Model file for the job. Use its own axes, mm. A direction names the side the tool comes from. Round coordinates to 2 decimals unless told otherwise and drop trailing zeros. Order: outer loops, then holes, each group sorted by start corner. A loop starts at its lowest first (then second) coordinate and runs counter-clockwise, first axis right, second up. Notation, with made-up numbers: M -2.75,85 L 38.25,85 A33 cw 38.25,119 Z; hole C 82.5,14 d2. An arc over 180 degrees is marked long. Return JSON: item names as keys, results as strings. Group by question number.
Item 1: Slice it at C-C on y = 9.75. Write the cut outline in (x, z), then the cut area to 3 significant figures.
Item 2: Pull direction X, two halves, no side cores. Call faces 1 (the face through (-1.743, 8.765, 1.901)), 2 (the face through (-7.374, 6.383, 2.322)), 3 (the face through (2, 11.112, 2)): pulls with the +X half, pulls with the -X half, needs draft (parallel to the pull), parting line crosses it, or undercut.
Item 3: Pin check, flat tips, straight feed: pin 1 Ø6 at (y, z) = (5, -4.5) entering from +X; pin 2 Ø4 at (x, z) = (0, -1) entering from -Y; pin 3 Ø6 at (x, y) = (-4.5, 2) entering from -Z. Stop position of each tip, or through.
Item 4: Slice it at D-D on y = 1.25. Write the cut outline in (x, z), then the cut area to 3 significant figures.
Item 5: Probe line 1 along X through (y, z) = (3.25, -2.75); line 2 along Z through (x, y) = (0, 7.55); line 3 along Y through (x, z) = (2.5, 2.5). List the from-to ranges inside material, lowest first.
Item 6: Which spindle directions (+Z, -Z, +X, -X, +Y, -Y) get a long thin tool onto all of the face, cutting with end or side? Do faces 4 (the face through (-1, 0, -4)), 5 (the face through (3.874, 3.219, 0.86)). Say none if no direction does.
Autodesk Inventor part; units mm, degrees
ref_plane "YZ Plane" through (0, 0, 0) normal (1, 0, 0) x (0, 1, 0)
ref_plane "XZ Plane" through (0, 0, 0) normal (0, 1, 0) x (-1, 0, 0)
ref_plane "XY Plane" through (0, 0, 0) normal (0, 0, 1) x (1, 0, 0)
sketch "Sketch1" plane through (0, 0, 0) normal (0, 1, 0) x (-1, 0, 0)
  circle A0 centre (0, 0) radius 7.9375
  dimension "d0" = 15.875
extrude "Extrusion1" add sketch "Sketch1" along normal blind 11.1125
sketch "Sketch2" plane through (0, 0, 0) normal (0, -1, 0) x (1, 0, 0)
  point P0 (0, 0)
  point P1 (0, 0)
hole "Hole1" at (0, 0, 0) direction (0, 1, 0) diameter 5.1594 end through all counterbore diameter 7.9375 counterbore depth 6.35
draft "FaceDraft1" angle 2.5 pull direction (0, -1, 0) faces at (-7.8347, 7.4083, -1.2733) fixed edges at (7.9375, 11.1125, 0)
fillet "Fillet1" radius 1.5875 1 edges at (7.4523, 0, 0)
properties part number "roundBumper" material "Rubber"
Output values:
{
 "1": {"outline": "C 0,0 d15.76; hole C 0,0 d5.16", "area": "174 mm²"},
 "2": {"face 1": "undercut", "face 2": "parting line crosses it", "face 3": "needs draft"},
 "3": {"pin 1": "x = 7.54", "pin 2": "y = 6.35", "pin 3": "z = -7.4"},
 "4": {"outline": "C 0,0 d14.97; hole C 0,0 d7.94", "area": "126 mm²"},
 "5": {"line 1": "-7.08 to -2.86, 2.86 to 7.08", "line 2": "-7.78 to -2.58, 2.58 to 7.78", "line 3": "6.35 to 11.11"},
 "6": {"face 4": "+Z, -Z, +X, -X, -Y", "face 5": "-Y"}
}
